```python
from build123d import *

# Parameters (mm, degrees)
SKETCH1_R           = 1.2
BOSS_EXTRUDE1_DEPTH = 2
SKETCH2_W           = 14
SKETCH2_H           = 14
BOSS_EXTRUDE2_DEPTH = 2


with BuildPart() as part:
    # Sketch1 → Boss-Extrude1 (new body)
    with BuildSketch(Plane.XY):
        with BuildLine():
            Line((58.085871194, -29), (79.085871194, -29))
            ThreePointArc((79.085871194, -29), (80.500084756, -29.585786438), (81.085871194, -31))
            Line((81.085871194, -31), (81.085871194, -52))
            ThreePointArc((81.085871194, -52), (80.500084756, -53.414213562), (79.085871194, -54))
            Line((79.085871194, -54), (58.085871194, -54))
            ThreePointArc((58.085871194, -54), (56.671657631, -53.414213562), (56.085871194, -52))
            Line((56.085871194, -52), (56.085871194, -31))
            ThreePointArc((56.085871194, -31), (56.671657631, -29.585786438), (58.085871194, -29))
        make_face()
        with Locations((58.085871194, -52)):
            Circle(SKETCH1_R, mode=Mode.SUBTRACT)
        with Locations((79.085871194, -52)):
            Circle(SKETCH1_R, mode=Mode.SUBTRACT)
        with Locations((79.085871194, -31)):
            Circle(SKETCH1_R, mode=Mode.SUBTRACT)
        with Locations((58.085871194, -31)):
            Circle(SKETCH1_R, mode=Mode.SUBTRACT)
    extrude(amount=BOSS_EXTRUDE1_DEPTH)

    # Sketch2 → Boss-Extrude2 (add)
    with BuildSketch(Plane.XY.offset(2)):
        with Locations((68.585871194, -41.5)):
            Rectangle(SKETCH2_W, SKETCH2_H)
    extrude(amount=BOSS_EXTRUDE2_DEPTH)


solid = part.part
```
Geometry check sheet. Reference: the model listing, model coordinates, mm. A direction names the side the tool comes from. Give positions to 0.01 mm unless a question says otherwise; leave off trailing zeros. Order: outer loops, then holes, each group sorted by start corner. A loop starts at its lowest first (then second) coordinate and runs counter-clockwise, first axis right, second up.
1. Section check D-D, the plane z = 3.55. Enter the section's corners in (x, y).
2. Section check B-B, the plane y = -37.25. Enter the section's corners in (x, z), and give its area (3 significant figures).
3. Access from +Z, -Z, +X, -X, +Y, -Y to the whole of each face (thin tool, end or side, straight path). Record for faces 1 (the face through (68, -48.5, 3)), 2 (the face through (61.586, -42, 3)), 3 (the face through (75.586, -42, 3)), 4 (the face through (68, -34.5, 3)).
4. Section check C-C, the plane z = 0.3. Enter the section's corners in (x, y).
5. Thickness scan on L1, parallel to Z at x = 78.5, y = -46.25; L2, parallel to X at y = -39.5, z = 2.1; L3, parallel to Y at x = 67.75, z = 2.55. Record the ranges inside material, lowest first.
6. Release check for a two-part mould opening along X. For faces 5 (the face through (59.23, -30.64, 0.99)), 6 (the face through (56.69, -53.43, 0.99)), 7 (the face through (69, -41, 0)), 8 (the face through (80.484, -29.57, 0.986)) record: pulls with the +X half, pulls with the -X half, needs draft (parallel to the pull), parting line crosses it, or undercut.
7. Section check A-A, the plane x = 62. Enter the section's corners in (y, z).
8. Gauge pin test, flat ends, axial feed: pin 1 Ø6 at (x, y) = (69, -33.5) entering from +Z; pin 2 Ø1.6 at (x, z) = (69.5, 3) entering from -Y; pin 3 Ø1 at (x, z) = (68.5, 3.5) entering from +Y. Record the tip position at first contact, or that the pin passes through.
Values follow:
1. outline: (61.59, -48.5) - (75.59, -48.5) - (75.59, -34.5) - (61.59, -34.5) - close
2. outline: (56.09, 0) - (81.09, 0) - (81.09, 2) - (75.59, 2) - (75.59, 4) - (61.59, 4) - (61.59, 2) - (56.09, 2) - close
2. area: 78.0 mm2
3. face 1: +Z, +X, -X, -Y
3. face 2: +Z, -X, +Y, -Y
3. face 3: +Z, +X, +Y, -Y
3. face 4: +Z, +X, -X, +Y
4. outline: (56.09, -52) arc R2 ccw to (58.09, -54) - (79.09, -54) arc R2 ccw to (81.09, -52) - (81.09, -31) arc R2 ccw to (79.09, -29) - (58.09, -29) arc R2 ccw to (56.09, -31) - close; hole circle Ø2.4 at (58.09, -52); hole circle Ø2.4 at (58.09, -31); hole circle Ø2.4 at (79.09, -52); hole circle Ø2.4 at (79.09, -31)
5. L1: z = 0 to 2
5. L2: x = 61.59 to 75.59
5. L3: y = -48.5 to -34.5
6. face 5: undercut
6. face 6: pulls with the -X half
6. face 7: needs draft
6. face 8: pulls with the +X half
7. outline: (-54, 0) - (-29, 0) - (-29, 2) - (-34.5, 2) - (-34.5, 4) - (-48.5, 4) - (-48.5, 2) - (-54, 2) - close
8. pin 1: stops at z = 4
8. pin 2: stops at y = -48.5
8. pin 3: stops at y = -34.5
